Can you work these out from the drawing? Everything is in mm from the part's minimum corner. A direction names the side the tool comes from. Give positions to 0.01 mm unless a question says otherwise; leave off trailing zeros. Write each loop counter-clockwise with the first axis right and the second up, starting at its lowest first coordinate (ties: lowest second). Pieces come first, ordered by that corner, then holes. Notation, with made-up numbers: (57.5, 26) -> (108.5, 26) arc R32 ccw to (108.5, 53) -> close; hole circle Ø11 at (34.25, 38). An arc over 180 degrees is marked (long way). Return JSON: item names as keys, results as strings.
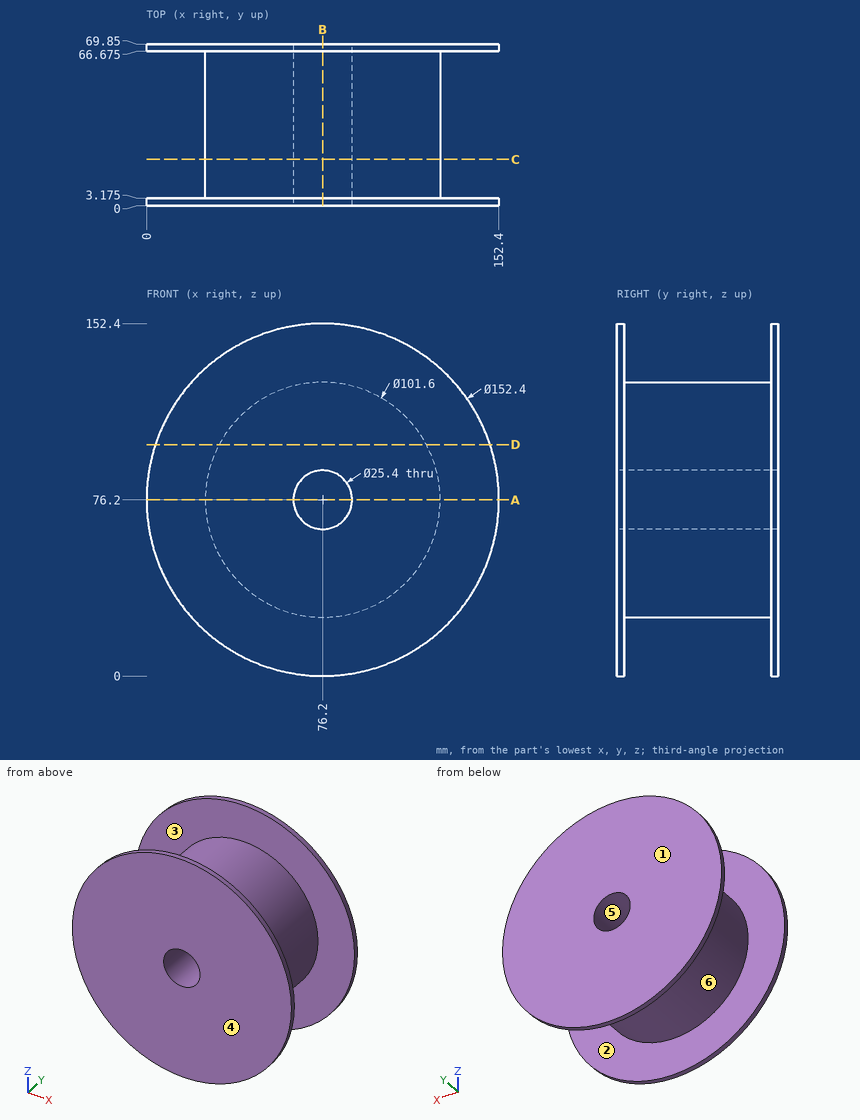
1. For pin 1 Ø8 at (y, z) = (58, 75.5) entering from +X; pin 2 Ø3 at (y, z) = (33.5, 83.5) entering from -X; pin 3 Ø10 at (y, z) = (58.5, 46) entering from -X; pin 4 Ø23 at (x, z) = (76.2, 76.2) entering from -Y, each with a flat end and sliding along its axis, tell me the tip position at first contact or that it passes through.
Taken from the geometry:
{"pin 1": "stops at x = 127", "pin 2": "stops at x = 25.73", "pin 3": "stops at x = 32.09", "pin 4": "passes through"}
2. Which directions (+Z, -Z, +X, -X, +Y, -Y) give clear straight access to the entire face, cutting with the end or side of a thin tool? Please do the marked faces 5 and 6.
Taken from the geometry:
{"face 5": "+Y, -Y", "face 6": "none"}
3. Suppose I cut it at C-C, the plane y = 20. List the corners of the cut face in (x, z) for me, and give its area (3 significant figures).
Taken from the geometry:
{"outline": "circle Ø101.6 at (76.2, 76.2); hole circle Ø25.4 at (76.2, 76.2)", "area": "7,600 mm²"}
4. If I drill on line 1 (Y direction, x = 112.5, z = 141) (3 decimals); line 2 (Z direction, x = 76.2, y = 16.5), over which ranges is the centre line in solid material (lowest first)? Write a range as [from, to].
Taken from the geometry:
{"line 1": "y = [0, 3.175], [66.675, 69.85]", "line 2": "z = [25.4, 63.5], [88.9, 127]"}
5. If we mould it in two halves opening along Y, with no side actions, what happens to the marked faces 1, 2, 3 and 4? For each: released by +Y, released by -Y, zero draft, split by the parting line, or undercut.
Taken from the geometry:
{"face 1": "released by +Y", "face 2": "undercut", "face 3": "undercut", "face 4": "released by -Y"}
6. Suppose I cut it at A-A, the plane z = 76.2. List the corners of the cut face in (x, y) for me (3 decimals), and give its area (3 significant figures).
Taken from the geometry:
{"outline": "(0, 0) -> (63.5, 0) -> (63.5, 69.85) -> (0, 69.85) -> (0, 66.675) -> (25.4, 66.675) -> (25.4, 3.175) -> (0, 3.175) -> close; (88.9, 0) -> (152.4, 0) -> (152.4, 3.175) -> (127, 3.175) -> (127, 66.675) -> (152.4, 66.675) -> (152.4, 69.85) -> (88.9, 69.85) -> close", "area": "5,650 mm²"}
7. Suppose I cut it at B-B, the plane x = 76.2. List the corners of the cut face in (y, z) for me (3 decimals).
Taken from the geometry:
{"outline": "(0, 0) -> (3.175, 0) -> (3.175, 25.4) -> (66.675, 25.4) -> (66.675, 0) -> (69.85, 0) -> (69.85, 63.5) -> (0, 63.5) -> close; (0, 88.9) -> (69.85, 88.9) -> (69.85, 152.4) -> (66.675, 152.4) -> (66.675, 127) -> (3.175, 127) -> (3.175, 152.4) -> (0, 152.4) -> close"}
8. Suppose I cut it at D-D, the plane z = 100. List the corners of the cut face in (x, y) for me (3 decimals), and give its area (3 significant figures).
Taken from the geometry:
{"outline": "(3.812, 0) -> (148.588, 0) -> (148.588, 3.175) -> (121.08, 3.175) -> (121.08, 66.675) -> (148.588, 66.675) -> (148.588, 69.85) -> (3.812, 69.85) -> (3.812, 66.675) -> (31.32, 66.675) -> (31.32, 3.175) -> (3.812, 3.175) -> close", "area": "6,620 mm²"}
